```python
from build123d import *

# Parameters (mm, degrees)
SKETCH2_R           = 8.25
SKETCH2_W           = 10
SKETCH2_H           = 10
BOSS_EXTRUDE1_DEPTH = 3.3
SKETCH3_R           = 9.45
SKETCH3_W           = 10
SKETCH3_H           = 10
BOSS_EXTRUDE2_DEPTH = 0.8
SKETCH4_R           = 7.65
CUT_EXTRUDE1_DEPTH  = 1.2
FILLET1_R           = 0.5


with BuildPart() as part:
    # Sketch2 → Boss-Extrude1 (new body)
    with BuildSketch(Plane.XY):
        Circle(SKETCH2_R)
        Rectangle(SKETCH2_W, SKETCH2_H, mode=Mode.SUBTRACT)
    extrude(amount=BOSS_EXTRUDE1_DEPTH)

    # Sketch3 → Boss-Extrude2 (add)
    with BuildSketch(Plane(origin=(0, 0, 0), x_dir=(-1, 0, 0), z_dir=(0, 0, -1))):
        Circle(SKETCH3_R)
        Rectangle(SKETCH3_W, SKETCH3_H, mode=Mode.SUBTRACT)
    extrude(amount=-BOSS_EXTRUDE2_DEPTH)

    # Sketch4 → Cut-Extrude1 (cut)
    with BuildSketch(Plane.XY.offset(3.3)):
        Circle(SKETCH4_R)
    extrude(amount=-CUT_EXTRUDE1_DEPTH, mode=Mode.SUBTRACT)

    # Fillet1
    fillet1_edges = [part.edges().sort_by_distance(p)[0] for p in [
        (9.45, 0, 0),
    ]]
    fillet(fillet1_edges, radius=FILLET1_R)


solid = part.part
```
Verification items for the finished model (mm, model axes). A direction names the side the tool comes from. Coordinates: 2 decimals unless noted, no trailing zeros. Loops run counter-clockwise (first coordinate to the right, second up) from the corner with the lowest first, then second, coordinate; pieces in that order, holes last. Notation, with made-up numbers: (-32.75, 14) - (9.25, 14) arc R19 ccw to (9.25, 26) - close; hole circle Ø6 at (73, 20.25). An arc over 180 degrees is marked (long way). Put each result on its own line as item: value.
Item 1: Set-up check for faces 1 (the face through (0, -6, 0)), 2 (the face through (0, -8.4, 0.8)), 3 (the face through (0, 5, 1)): record each of +Z, -Z, +X, -X, +Y, -Y from which the full face is reachable in a straight line by a thin tool's end or side.
Conclusion:
face 1: -Z, +X, -X, +Y, -Y
face 2: +Z
face 3: +Z, -Z
Item 2: Gauge pin test, flat ends, axial feed: pin 1 Ø5 at (x, y) = (-6.5, 0) entering from -Z; pin 2 Ø1.7 at (y, z) = (-2, 1.5) entering from -X; pin 3 Ø0.6 at (x, z) = (-1, 0.5) entering from -Y; pin 4 Ø3 at (x, y) = (0, 3) entering from -Z. Record the tip position at first contact, or that the pin passes through.
Conclusion:
pin 1: stops at z = 0
pin 2: stops at x = -9.33
pin 3: stops at y = -9.42
pin 4: passes through
Item 3: Draft check along X on faces 4 (the face through (1.23, 9.37, 0.65)), 5 (the face through (5, -6, 3.3)), 6 (the face through (-1.658, -7.468, 2.708)), 7 (the face through (0, -5, 1)). Enter one of: pulls with the +X half, pulls with the -X half, needs draft (parallel to the pull), parting line crosses it, or undercut.
Conclusion:
face 4: parting line crosses it
face 5: needs draft
face 6: undercut
face 7: undercut
Item 4: Section check A-A (x = 0). Enter the section's corners in (y, z), then the cut area to 3 significant figures.
Conclusion:
outline: (-9.45, 0.5) arc R0.5 ccw to (-8.95, 0) - (-5, 0) - (-5, 2.1) - (-7.65, 2.1) - (-7.65, 3.3) - (-8.25, 3.3) - (-8.25, 0.8) - (-9.45, 0.8) - close; (5, 0) - (8.95, 0) arc R0.5 ccw to (9.45, 0.5) - (9.45, 0.8) - (8.25, 0.8) - (8.25, 3.3) - (7.65, 3.3) - (7.65, 2.1) - (5, 2.1) - close
area: 16.9 mm2
Item 5: Section check C-C (z = 1.75). Enter the section's corners in (x, y).
Conclusion:
outline: circle Ø16.5 at (0, 0); hole (-5, -5) - (5, -5) - (5, 5) - (-5, 5) - close
Item 6: Scan lines: line 1 along Y through (x, z) = (0, 2.55); line 2 along Z through (x, y) = (-4, 7.25); line 3 along Z through (x, y) = (6.5, -1.75). Record each from-to range of solid material in increasing order.
Conclusion:
line 1: y = -8.25 to -7.65, 7.65 to 8.25
line 2: z = 0 to 0.8
line 3: z = 0 to 2.1
